from build123d import *

# Parameters (mm, degrees)
F2_R = 0.762
F4_D = 7.9375


with BuildPart() as f1:
    # F0 (on Front) → F1 (revolve)
    with BuildSketch(Plane.XZ):
        Polygon((9.525, 0), (0, 0), (0, -19.05), (7.9375, -19.05), (7.9375, -3.175), (9.525, -3.175), align=None)
    revolve(axis=Axis((0, 0, -9.525), (0, 0, -1)))

    # F2
    f2_edges = [f1.edges().sort_by_distance(p)[0] for p in [
        (-9.525, 0, 0),
    ]]
    fillet(f2_edges, radius=F2_R)

    # F4 (through all)
    with Locations(Plane.XY):
        with Locations((0, 0)):
            Hole(F4_D / 2)


solid = f1.part
Model file for the job. Use its own axes, mm. A direction names the side the tool comes from. Give positions to 0.01 mm unless a question says otherwise; leave off trailing zeros. Order: outer loops, then holes, each group sorted by start corner. A loop starts at its lowest first (then second) coordinate and runs counter-clockwise, first axis right, second up. Notation, with made-up numbers: (13.25, 8.25) - (39.25, 8.25) arc R27 cw to (39.25, 24.25) - close; hole circle Ø9 at (61.25, 85.5). An arc over 180 degrees is marked (long way). Return JSON: item names as keys, results as strings.
1) Pull direction Y, two halves, no side cores. Call faces 1 (the cylindrical face through (0.86, -3.874, -9.658)), 2 (the flat face through (2, -8, -3.175)), 3 (the cylindrical face through (-7.559, 5.796, -1.952)): pulls with the +Y half, pulls with the -Y half, needs draft (parallel to the pull), parting line crosses it, or undercut.
Geometry says:
{"face 1": "undercut", "face 2": "needs draft", "face 3": "parting line crosses it"}
2) Cut at C-C, the plane z = -9.5. Give the cut face in (x, y) (1 decimal).
Geometry says:
{"outline": "circle Ø15.9 at (0, 0); hole circle Ø7.9 at (0, 0)"}
3) Probe line 1 (Y direction, x = 0, z = -11); line 2 (Z direction, x = -8, y = -2) (3 decimals); line 3 (Y direction, x = 3.5, z = -12.75). List the from-to ranges inside material, lowest first. Write a range as from..to.
Geometry says:
{"line 1": "-7.94..-3.97, 3.97..7.94", "line 2": "-3.175..0", "line 3": "-7.12..-1.87, 1.87..7.12"}
4) Flat gauge pins, fed straight in: P1, Ø1, axis at x = 1, z = -9, coming from the +Y side; P2, Ø6.5, axis at x = 0, y = 0, coming from the -Z side; P3, Ø8, axis at x = 7, z = -6, coming from the -Y side; P4, Ø1, axis at x = 5.5, z = -13.5, coming from the +Y side. Where does each tip first touch, or does it go through?
Geometry says:
{"P1": "y = 7.92", "P2": "through", "P3": "y = -8.56", "P4": "y = 6.16"}
5) 3-axis set-ups, long thin cutter, end or side, ignore diameter. For faces 4 (the flat face through (4, 2, 0)), 5 (the cylindrical face through (-1.72, 7.75, -11)): which of +Z, -Z, +X, -X, +Y, -Y reach the whole face in a straight line?
Geometry says:
{"face 4": "+Z, +X, -X, +Y, -Y", "face 5": "-Z"}
